Autodesk Inventor part; units mm, degrees
ref_plane "YZ Plane" through (0, 0, 0) normal (1, 0, 0) x (0, 1, 0)
ref_plane "XZ Plane" through (0, 0, 0) normal (0, 1, 0) x (-1, 0, 0)
ref_plane "XY Plane" through (0, 0, 0) normal (0, 0, 1) x (1, 0, 0)
sketch "Sketch1" plane through (0, 0, 0) normal (0, 1, 0) x (-1, 0, 0)
  line L0 (-71.5, -85) -> (71.5, -85)
  line L1 (71.5, -85) -> (71.5, 85)
  line L2 (71.5, 85) -> (-71.5, 85)
  line L3 (-71.5, 85) -> (-71.5, -85)
  line L4 (-71.5, -85) -> (71.5, 85) construction
  line L5 (71.5, -85) -> (-71.5, 85) construction
  point P0 (0, 0)
  dimension "d0" = 143
  dimension "d1" = 170
extrude "Base" add sketch "Sketch1" along normal blind 23
sketch "Sketch2" plane through (0, 0, 0) normal (0, -1, 0) x (1, 0, 0)
  line L0 (-60, -72.5) -> (60, -72.5)
  line L1 (60, -72.5) -> (60, 72.5)
  line L2 (60, 72.5) -> (-60, 72.5)
  line L3 (-60, 72.5) -> (-60, -72.5)
  line L4 (-60, -72.5) -> (60, 72.5) construction
  line L5 (60, -72.5) -> (-60, 72.5) construction
  point P0 (0, 0)
  dimension "d4" = 120
  dimension "d5" = 145
extrude "Extrusion2" cut sketch "Sketch2" against normal through all
sketch "Sketch3" plane through (0, 0, 0) normal (0, -1, 0) x (1, 0, 0)
  line L0 (63.65, -75.5) -> (-63.65, -75.5)
  line L1 (-63.65, -75.5) -> (-63.65, 75.5)
  line L2 (-63.65, 75.5) -> (63.65, 75.5)
  line L3 (63.65, 75.5) -> (63.65, -75.5)
  line L4 (-60, 72.5) -> (60, 72.5)
  line L5 (-60, -72.5) -> (-60, 72.5)
  line L6 (68.85, -80.7) -> (-68.85, -80.7)
  line L7 (-68.85, -80.7) -> (-68.85, 80.7)
  line L8 (-68.85, 80.7) -> (68.85, 80.7)
  line L9 (68.85, 80.7) -> (68.85, -80.7)
  line L10 (-71.5, 85) -> (71.5, 85)
  point P0 (0, 0)
  point P1 (63.65, 0)
  point P2 (68.85, 0)
  dimension "d9" = 3.65
  dimension "d10" = 5.2
  dimension "d11" = 12.5
  dimension "d38" = 5.2
  dimension "d39" = 151
extrude "Extrusion3" cut sketch "Sketch3" against normal blind 12
sketch "Sketch4" plane through (0, 12, 0) normal (0, -1, 0) x (1, 0, 0)
  line L0 (-68.85, 80.7) -> (68.85, 80.7)
  line L1 (63.65, 75.5) -> (-63.65, 75.5)
  line L2 (-53.85, 80.7) -> (-41.85, 80.7)
  line L3 (-41.85, 80.7) -> (-41.85, 75.5)
  line L4 (-41.85, 75.5) -> (-53.85, 75.5)
  line L5 (-53.85, 75.5) -> (-53.85, 80.7)
  line L6 (-68.85, -80.7) -> (-68.85, 80.7)
  line L7 (-63.65, 75.5) -> (-63.65, -75.5)
  line L8 (-63.65, 66.4) -> (-68.85, 66.4)
  line L9 (-68.85, 66.4) -> (-68.85, 54.4)
  line L10 (-68.85, 54.4) -> (-63.65, 54.4)
  line L11 (-63.65, 54.4) -> (-63.65, 66.4)
  line L12 (63.65, -75.5) -> (63.65, 75.5)
  line L13 (68.85, 80.7) -> (68.85, -80.7)
  line L14 (63.65, 66.4) -> (68.85, 66.4)
  line L15 (68.85, 66.4) -> (68.85, 54.4)
  line L16 (68.85, 54.4) -> (63.65, 54.4)
  line L17 (63.65, 54.4) -> (63.65, 66.4)
  line L18 (-63.65, -75.5) -> (63.65, -75.5)
  line L19 (68.85, -80.7) -> (-68.85, -80.7)
  line L20 (-53.85, -75.5) -> (-41.85, -75.5)
  line L21 (-41.85, -75.5) -> (-41.85, -80.7)
  line L22 (-41.85, -80.7) -> (-53.85, -80.7)
  line L23 (-53.85, -80.7) -> (-53.85, -75.5)
  line L24 (-68.85, -66.4) -> (-63.65, -66.4)
  line L25 (-63.65, -66.4) -> (-63.65, -54.4)
  line L26 (-63.65, -54.4) -> (-68.85, -54.4)
  line L27 (-68.85, -54.4) -> (-68.85, -66.4)
  line L28 (53.85, -80.7) -> (41.85, -80.7)
  line L29 (41.85, -80.7) -> (41.85, -75.5)
  line L30 (41.85, -75.5) -> (53.85, -75.5)
  line L31 (53.85, -75.5) -> (53.85, -80.7)
  line L32 (68.85, -54.4) -> (63.65, -54.4)
  line L33 (63.65, -54.4) -> (63.65, -66.4)
  line L34 (63.65, -66.4) -> (68.85, -66.4)
  line L35 (68.85, -66.4) -> (68.85, -54.4)
  line L36 (53.85, 75.5) -> (41.85, 75.5)
  line L37 (41.85, 75.5) -> (41.85, 80.7)
  line L38 (41.85, 80.7) -> (53.85, 80.7)
  line L39 (53.85, 80.7) -> (53.85, 75.5)
  point P0 (0, 0)
  point P1 (66.25, 66.4)
  point P2 (-66.25, 66.4)
  point P3 (-53.85, -78.1)
  point P4 (-53.85, 78.1)
  point P5 (66.25, -54.4)
  point P6 (-66.25, -54.4)
  point P7 (41.85, 78.1)
  point P8 (41.85, -78.1)
  dimension "d14" = 12
  dimension "d15" = 15
  dimension "d16" = 12
  dimension "d17" = 14.3
  dimension "d18" = 12
  dimension "d19" = 12
  dimension "d20" = 14.3
  dimension "d21" = 12
  dimension "d22" = 12
  dimension "d23" = 15
  dimension "d24" = 12
  dimension "d25" = 12
extrude "Extrusion4" add sketch "Sketch4" along normal blind 7 contours L0 L3 L1 L5 | L8 L7 L10 L6 | L0 L39 L1 L37 | L26 L7 L24 L6 | L13 L16 L12 L14 | L23 L18 L21 L19 | L13 L34 L12 L32 | L29 L18 L31 L19
fillet "Fillet1" radius 1.25 16 edges at (-66.25, 5, 54.4) (-66.25, 5, 66.4) (-66.25, 5, -66.4) (-66.25, 5, -54.4) (66.25, 5, -66.4) (66.25, 5, -54.4) (66.25, 5, 54.4) (66.25, 5, 66.4) (53.85, 5, -78.1) (41.85, 5, -78.1) (-53.85, 5, -78.1) (-41.85, 5, -78.1) (-53.85, 5, 78.1) (-41.85, 5, 78.1) (41.85, 5, 78.1) (53.85, 5, 78.1)
sketch "Sketch5" plane through (71.5, 0, -85) normal (0, 0, -1) x (-1, 0, 0)
  line L0 (71.5, 0) -> (71.5, 23) construction
  line L1 (131.5, 23) -> (11.5, 23) construction
  line L2 (5, 20.05) -> (138, 20.05)
  line L3 (138, 20.05) -> (138, 14.8)
  line L4 (138, 14.8) -> (5, 14.8)
  line L5 (5, 14.8) -> (5, 20.05)
  line L6 (0, 0) -> (143, 0)
  point P0 (71.5, 20.05)
  dimension "d29" = 133
  dimension "d30" = 5.25
  dimension "d31" = 14.8
extrude "Extrusion5" cut sketch "Sketch5" against normal blind 165
fillet "Fillet2" radius 3 2 edges at (71.5, 23, 0) (-71.5, 23, 0)
sketch "Sketch6" plane through (71.5, 0, -85) normal (0, 0, -1) x (-1, 0, 0)
  line L0 (3, 23) -> (140, 23)
  line L1 (5, 20.05) -> (138, 20.05)
  line L2 (11.5, 23) -> (131.5, 23)
  line L3 (131.5, 23) -> (131.5, 20.05)
  line L4 (131.5, 20.05) -> (11.5, 20.05)
  line L5 (11.5, 20.05) -> (11.5, 23)
  line L6 (0, 0) -> (143, 0) construction
  point P0 (71.5, 0)
  point P1 (71.5, 23)
  point P2 (71.5, 0)
  dimension "d35" = 120
extrude "Extrusion6" cut sketch "Sketch6" against normal blind 12.5
equation "\"d9\" = d8"
equation "\"d16\" = d14"
equation "\"d18\" = d14"
equation "\"d19\" = d14"
equation "\"d20\" = d17"
equation "\"d21\" = d19"
equation "\"d22\" = d14"
equation "\"d23\" = d15"
equation "\"d24\" = d14"
equation "\"d8\" = -0.5 * d10 + 0.5 * d11"
properties part number "top_bracket_for_5mm"
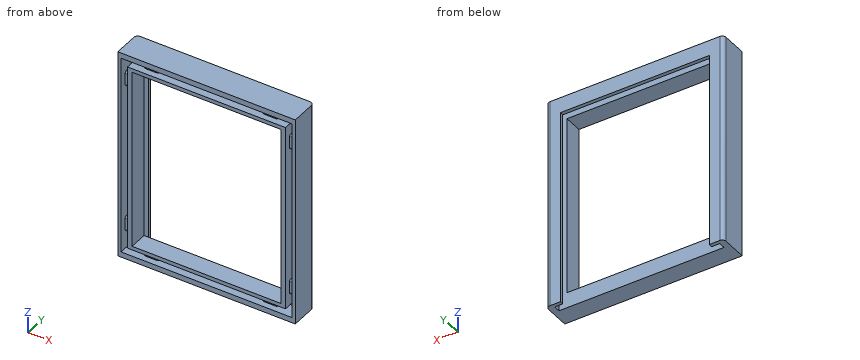
Build history of the part. All positions in model axes, mm. Coordinates: 2 decimals unless noted, no trailing zeros. Order: outer loops, then holes, each group sorted by start corner. A loop starts at its lowest first (then second) coordinate and runs counter-clockwise, first axis right, second up. Notation, with made-up numbers: (9.25, -20.75) - (49.25, -20.75) arc R24 cw to (49.25, 14.25) - close; hole circle Ø7 at (-3.75, -3). An arc over 180 degrees is marked (long way). Put each result on its own line as item: value.
1. Drop flat-ended pins along their axis: P1, Ø2.5, axis at y = 21.5, z = -19.5, coming from the -X side; P2, Ø1.6, axis at x = -67, z = 62.5, coming from the -Y side. Give the stop position or say it passes through.
Answer sheet:
P1: stops at x = -71.49
P2: stops at y = 5
2. Saw through at B-B (z = 2). Write the cut outline in (x, y), and give its area (3 significant figures).
Answer sheet:
outline: (-71.5, 0) - (-68.85, 0) - (-68.85, 12) - (-63.65, 12) - (-63.65, 0) - (-60, 0) - (-60, 14.8) - (-66.5, 14.8) - (-66.5, 20.05) - (-60, 20.05) - (-60, 23) - (-68.5, 23) arc R3 ccw to (-71.5, 20) - close; (60, 0) - (63.65, 0) - (63.65, 12) - (68.85, 12) - (68.85, 0) - (71.5, 0) - (71.5, 20) arc R3 ccw to (68.5, 23) - (60, 23) - (60, 20.05) - (66.5, 20.05) - (66.5, 14.8) - (60, 14.8) - close
area: 332 mm^2
3. Saw through at A-A (y = 2.5). Write the cut outline in (x, z).
Answer sheet:
outline: (-71.5, -85) - (71.5, -85) - (71.5, 85) - (-71.5, 85) - close; (-63.65, -75.5) - (63.65, -75.5) - (63.65, 75.5) - (-63.65, 75.5) - close; hole (-68.85, -80.7) - (68.85, -80.7) - (68.85, 80.7) - (-68.85, 80.7) - close; hole (-60, -72.5) - (60, -72.5) - (60, 72.5) - (-60, 72.5) - close
4. Saw through at C-C (x = 19.5). Write the cut outline in (y, z), and give its area (3 significant figures).
Answer sheet:
outline: (0, -85) - (14.8, -85) - (14.8, -72.5) - (0, -72.5) - (0, -75.5) - (12, -75.5) - (12, -80.7) - (0, -80.7) - close; (0, 72.5) - (14.8, 72.5) - (14.8, 80) - (20.05, 80) - (20.05, 72.5) - (23, 72.5) - (23, 85) - (0, 85) - (0, 80.7) - (12, 80.7) - (12, 75.5) - (0, 75.5) - close
area: 308 mm^2
5. Saw through at D-D (y = 16.75). Write the cut outline in (x, z), and give its area (4 significant figures).
Answer sheet:
outline: (-71.5, -85) - (-66.5, -85) - (-66.5, 80) - (66.5, 80) - (66.5, -85) - (71.5, -85) - (71.5, 85) - (-71.5, 85) - close
area: 2,365 mm^2
6. Probe line 1 along Z through (x, y) = (-35, 7); line 2 along X through (y, z) = (11.25, 12.5); line 3 along Z through (x, y) = (-51, 6). List the from-to ranges inside material, lowest first. Write a range as [from, to].
Answer sheet:
line 1: z = [-85, -80.7], [-75.5, -72.5], [72.5, 75.5], [80.7, 85]
line 2: x = [-71.5, -68.85], [-63.65, -60], [60, 63.65], [68.85, 71.5]
line 3: z = [-85, -72.5], [72.5, 85]
